Geometry: final body of the model. Coordinates: model frame, mm. A direction names the side the tool comes from. Give positions to 0.01 mm unless a question says otherwise; leave off trailing zeros. Order: outer loops, then holes, each group sorted by start corner. A loop starts at its lowest first (then second) coordinate and runs counter-clockwise, first axis right, second up. Notation, with made-up numbers: (41, 6.5) -> (65, 6.5) arc R21 ccw to (65, 41.5) -> close; hole circle Ø2 at (23.5, 20.5). An arc over 180 degrees is marked (long way). One line per question, with ' | ' between items.
from build123d import *

# Parameters (mm, degrees)
F1_DEPTH   = 650
F2_W       = 75
F2_H       = 40
F3_DEPTH   = 8
F5_D       = 8
F5_ON_F2_D = 8
F6_D       = 10


with BuildPart() as f1:
    # F0 (on Front) → F1 (new body, symmetric)
    with BuildSketch(Plane.XZ):
        Polygon((21, -20), (25, -20), (25, 20), (-25, 20), (-25, -20), (-21, -20), (-21, 16), (21, 16), align=None)
    extrude(amount=F1_DEPTH, both=True)

    # F2 (on face) → F3 (cut)
    with BuildSketch(Plane.YZ.offset(25)):
        with Locations((-612.5, 0)):
            Rectangle(F2_W, F2_H)
        with Locations((612.5, 0)):
            Rectangle(F2_W, F2_H)
    extrude(amount=-F3_DEPTH, mode=Mode.SUBTRACT)

    # F5 (through all)
    with Locations(Plane.XY.offset(20)):
        with Locations((7, -625), (7, -640), (7, 640), (7, 625)):
            Hole(F5_D / 2)

    # F5 on F2 (through all)
    with Locations(Plane.YZ.offset(25)):
        with Locations((-565, -2), (-545, -2), (565, -2), (545, -2)):
            Hole(F5_ON_F2_D / 2)

    # F6 (through all)
    with Locations(Plane.XY.offset(20)):
        with Locations((2.25, -590), (2.25, 590)):
            Hole(F6_D / 2)


solid = f1.part
1) Material intervals for probe 1 along X at (y, z) = (590, 17); probe 2 along X at (y, z) = (640, 17.45); probe 3 along Z at (x, y) = (-22, -565), sorted ascending. Write a range as from..to.
Check result:
probe 1: x = -25..-2.75, 7.25..17 | probe 2: x = -25..3, 11..17 | probe 3: z = -20..-6, 2..20
2) Pull-direction query (X, two-part tool) for faces 3 (the flat face through (0, -9, 20)), 4 (the flat face through (25, -8, 0)), 5 (the flat face through (-21, -9, -2)); classes: +X half, -X half, draft (parallel to the pull), parting line (faces both ways), or undercut.
Check result:
face 3: draft | face 4: +X half | face 5: undercut
3) Section B-B on x = -10.5. Return loops of the section in (y, z).
Check result:
outline: (-650, 16) -> (650, 16) -> (650, 20) -> (-650, 20) -> close
4) Contact query for flat-ended pins moving along their axis: pin 1 Ø4.5 at (y, z) = (-622.5, 18) entering from +X; pin 2 Ø2 at (x, y) = (2, -283) entering from -Z; pin 3 Ø13 at (y, z) = (545, -2) entering from -X; pin 4 Ø4 at (x, z) = (22.5, -10) entering from +Y. Output: stop coordinate, or through.
Check result:
pin 1: stops at x = 17 | pin 2: stops at z = 16 | pin 3: stops at x = -25 | pin 4: stops at y = 575
5) Section A-A on y = -104. Return loops of the section in (x, z).
Check result:
outline: (-25, -20) -> (-21, -20) -> (-21, 16) -> (21, 16) -> (21, -20) -> (25, -20) -> (25, 20) -> (-25, 20) -> close
6) Set-up query: faces 1 (the flat face through (21, -8, -2)), 2 (the flat face through (-21.2, 650, 9)). Return all of +Z, -Z, +X, -X, +Y, -Y with unobstructed straight access to the full face (end or side cutting, diameter ignored); none if empty.
Check result:
face 1: -Z, +Y, -Y | face 2: +Z, -Z, +X, -X, +Y
